For this review, take the finished solid that the model builds, in its own axes (mm). Coordinates: 2 decimals unless noted, no trailing zeros. Loops run counter-clockwise (first coordinate to the right, second up) from the corner with the lowest first, then second, coordinate; pieces in that order, holes last. Notation, with made-up numbers: (4, -30) -> (43, -30) arc R5 ccw to (43, -26) -> close; hole circle Ø2 at (34, -4.5). An arc over 180 degrees is marked (long way). One line per item, written item: value.
from build123d import *

# Parameters (mm, degrees)
SKETCH1_R           = 14.2875
SKETCH1_R_2         = 9.525
SKETCH1_R_3         = 2.4892
BOSS_EXTRUDE3_DEPTH = 3.175


with BuildPart() as part:
    # Sketch1 → Boss-Extrude3 (new body)
    with BuildSketch(Plane.XY):
        Polygon((93.273189322, 200.025), (-25.168955849, -53.975), (-25.168955849, -117.475), (279.631044151, -117.475), (279.631044151, -53.975), (398.073189322, 200.025), align=None)
        with Locations((32.394386098, 20.6375)):
            Circle(SKETCH1_R, mode=Mode.SUBTRACT)
        with Locations((137.394386098, 20.6375)):
            Circle(SKETCH1_R, mode=Mode.SUBTRACT)
        with Locations((242.394386098, 20.6375)):
            Circle(SKETCH1_R, mode=Mode.SUBTRACT)
        with Locations((106.42072683, 179.3875)):
            Circle(SKETCH1_R, mode=Mode.SUBTRACT)
        with Locations((211.39892683, 179.3875)):
            Circle(SKETCH1_R, mode=Mode.SUBTRACT)
        with Locations((189.894386098, -18.746667191)):
            Circle(SKETCH1_R_2, mode=Mode.SUBTRACT)
        with Locations((84.894386098, -21.788906871)):
            Circle(SKETCH1_R_2, mode=Mode.SUBTRACT)
        with Locations((266.931044151, -79.375)):
            Circle(SKETCH1_R_3, mode=Mode.SUBTRACT)
        with Locations((-12.468955849, -104.775)):
            Circle(SKETCH1_R_3, mode=Mode.SUBTRACT)
        with Locations((0.231044151, -104.775)):
            Circle(SKETCH1_R_3, mode=Mode.SUBTRACT)
        with Locations((12.931044151, -104.775)):
            Circle(SKETCH1_R_3, mode=Mode.SUBTRACT)
        with Locations((25.631044151, -104.775)):
            Circle(SKETCH1_R_3, mode=Mode.SUBTRACT)
        with Locations((-12.468955849, -92.075)):
            Circle(SKETCH1_R_3, mode=Mode.SUBTRACT)
        with Locations((0.231044151, -92.075)):
            Circle(SKETCH1_R_3, mode=Mode.SUBTRACT)
        with Locations((-12.468955849, -79.375)):
            Circle(SKETCH1_R_3, mode=Mode.SUBTRACT)
        with Locations((0.231044151, -79.375)):
            Circle(SKETCH1_R_3, mode=Mode.SUBTRACT)
        with Locations((12.931044151, -92.075)):
            Circle(SKETCH1_R_3, mode=Mode.SUBTRACT)
        with Locations((25.631044151, -92.075)):
            Circle(SKETCH1_R_3, mode=Mode.SUBTRACT)
        with Locations((12.931044151, -79.375)):
            Circle(SKETCH1_R_3, mode=Mode.SUBTRACT)
        with Locations((25.631044151, -79.375)):
            Circle(SKETCH1_R_3, mode=Mode.SUBTRACT)
        with Locations((38.331044151, -104.775)):
            Circle(SKETCH1_R_3, mode=Mode.SUBTRACT)
        with Locations((51.031044151, -104.775)):
            Circle(SKETCH1_R_3, mode=Mode.SUBTRACT)
        with Locations((63.731044151, -104.775)):
            Circle(SKETCH1_R_3, mode=Mode.SUBTRACT)
        with Locations((76.431044151, -104.775)):
            Circle(SKETCH1_R_3, mode=Mode.SUBTRACT)
        with Locations((38.331044151, -92.075)):
            Circle(SKETCH1_R_3, mode=Mode.SUBTRACT)
        with Locations((51.031044151, -92.075)):
            Circle(SKETCH1_R_3, mode=Mode.SUBTRACT)
        with Locations((38.331044151, -79.375)):
            Circle(SKETCH1_R_3, mode=Mode.SUBTRACT)
        with Locations((51.031044151, -79.375)):
            Circle(SKETCH1_R_3, mode=Mode.SUBTRACT)
        with Locations((63.731044151, -92.075)):
            Circle(SKETCH1_R_3, mode=Mode.SUBTRACT)
        with Locations((76.431044151, -92.075)):
            Circle(SKETCH1_R_3, mode=Mode.SUBTRACT)
        with Locations((63.731044151, -79.375)):
            Circle(SKETCH1_R_3, mode=Mode.SUBTRACT)
        with Locations((76.431044151, -79.375)):
            Circle(SKETCH1_R_3, mode=Mode.SUBTRACT)
        with Locations((89.131044151, -104.775)):
            Circle(SKETCH1_R_3, mode=Mode.SUBTRACT)
        with Locations((101.831044151, -104.775)):
            Circle(SKETCH1_R_3, mode=Mode.SUBTRACT)
        with Locations((114.531044151, -104.775)):
            Circle(SKETCH1_R_3, mode=Mode.SUBTRACT)
        with Locations((127.231044151, -104.775)):
            Circle(SKETCH1_R_3, mode=Mode.SUBTRACT)
        with Locations((89.131044151, -92.075)):
            Circle(SKETCH1_R_3, mode=Mode.SUBTRACT)
        with Locations((101.831044151, -92.075)):
            Circle(SKETCH1_R_3, mode=Mode.SUBTRACT)
        with Locations((89.131044151, -79.375)):
            Circle(SKETCH1_R_3, mode=Mode.SUBTRACT)
        with Locations((101.831044151, -79.375)):
            Circle(SKETCH1_R_3, mode=Mode.SUBTRACT)
        with Locations((114.531044151, -92.075)):
            Circle(SKETCH1_R_3, mode=Mode.SUBTRACT)
        with Locations((127.231044151, -92.075)):
            Circle(SKETCH1_R_3, mode=Mode.SUBTRACT)
        with Locations((114.531044151, -79.375)):
            Circle(SKETCH1_R_3, mode=Mode.SUBTRACT)
        with Locations((127.231044151, -79.375)):
            Circle(SKETCH1_R_3, mode=Mode.SUBTRACT)
        with Locations((139.931044151, -104.775)):
            Circle(SKETCH1_R_3, mode=Mode.SUBTRACT)
        with Locations((152.631044151, -104.775)):
            Circle(SKETCH1_R_3, mode=Mode.SUBTRACT)
        with Locations((165.331044151, -104.775)):
            Circle(SKETCH1_R_3, mode=Mode.SUBTRACT)
        with Locations((178.031044151, -104.775)):
            Circle(SKETCH1_R_3, mode=Mode.SUBTRACT)
        with Locations((139.931044151, -92.075)):
            Circle(SKETCH1_R_3, mode=Mode.SUBTRACT)
        with Locations((152.631044151, -92.075)):
            Circle(SKETCH1_R_3, mode=Mode.SUBTRACT)
        with Locations((139.931044151, -79.375)):
            Circle(SKETCH1_R_3, mode=Mode.SUBTRACT)
        with Locations((152.631044151, -79.375)):
            Circle(SKETCH1_R_3, mode=Mode.SUBTRACT)
        with Locations((165.331044151, -92.075)):
            Circle(SKETCH1_R_3, mode=Mode.SUBTRACT)
        with Locations((178.031044151, -92.075)):
            Circle(SKETCH1_R_3, mode=Mode.SUBTRACT)
        with Locations((165.331044151, -79.375)):
            Circle(SKETCH1_R_3, mode=Mode.SUBTRACT)
        with Locations((178.031044151, -79.375)):
            Circle(SKETCH1_R_3, mode=Mode.SUBTRACT)
        with Locations((190.731044151, -104.775)):
            Circle(SKETCH1_R_3, mode=Mode.SUBTRACT)
        with Locations((203.431044151, -104.775)):
            Circle(SKETCH1_R_3, mode=Mode.SUBTRACT)
        with Locations((216.131044151, -104.775)):
            Circle(SKETCH1_R_3, mode=Mode.SUBTRACT)
        with Locations((228.831044151, -104.775)):
            Circle(SKETCH1_R_3, mode=Mode.SUBTRACT)
        with Locations((190.731044151, -92.075)):
            Circle(SKETCH1_R_3, mode=Mode.SUBTRACT)
        with Locations((203.431044151, -92.075)):
            Circle(SKETCH1_R_3, mode=Mode.SUBTRACT)
        with Locations((190.731044151, -79.375)):
            Circle(SKETCH1_R_3, mode=Mode.SUBTRACT)
        with Locations((203.431044151, -79.375)):
            Circle(SKETCH1_R_3, mode=Mode.SUBTRACT)
        with Locations((216.131044151, -92.075)):
            Circle(SKETCH1_R_3, mode=Mode.SUBTRACT)
        with Locations((228.831044151, -92.075)):
            Circle(SKETCH1_R_3, mode=Mode.SUBTRACT)
        with Locations((216.131044151, -79.375)):
            Circle(SKETCH1_R_3, mode=Mode.SUBTRACT)
        with Locations((228.831044151, -79.375)):
            Circle(SKETCH1_R_3, mode=Mode.SUBTRACT)
        with Locations((241.531044151, -104.775)):
            Circle(SKETCH1_R_3, mode=Mode.SUBTRACT)
        with Locations((254.231044151, -104.775)):
            Circle(SKETCH1_R_3, mode=Mode.SUBTRACT)
        with Locations((266.931044151, -104.775)):
            Circle(SKETCH1_R_3, mode=Mode.SUBTRACT)
        with Locations((241.531044151, -92.075)):
            Circle(SKETCH1_R_3, mode=Mode.SUBTRACT)
        with Locations((254.231044151, -92.075)):
            Circle(SKETCH1_R_3, mode=Mode.SUBTRACT)
        with Locations((241.531044151, -79.375)):
            Circle(SKETCH1_R_3, mode=Mode.SUBTRACT)
        with Locations((254.231044151, -79.375)):
            Circle(SKETCH1_R_3, mode=Mode.SUBTRACT)
        with Locations((266.931044151, -92.075)):
            Circle(SKETCH1_R_3, mode=Mode.SUBTRACT)
    extrude(amount=BOSS_EXTRUDE3_DEPTH)


solid = part.part
1. Take a section at C-C, the plane z = 0.55. Give the number of separate pieces and of enclosed holes in the cut face, and give its area (3 significant figures).
Return value:
separate pieces: 1
enclosed holes: 76
area: 91,700 mm2
2. To check wall thickness, follow probe 1 along Y at (x, z) = (178, 0.7) (3 decimals); probe 2 along Y at (x, z) = (78, 1.15) (3 decimals); probe 3 along Y at (x, z) = (13.5, 2.95) (3 decimals). State the ranges of each line that lie inside material, in increasing order. Write a range as from..to.
Return value:
probe 1: y = -117.475..-107.264, -102.286..-94.564, -89.586..-81.864, -76.886..200.025
probe 2: y = -117.475..-106.707, -102.843..-94.007, -90.143..-81.307, -77.443..-28.361, -15.217..167.272
probe 3: y = -117.475..-107.198, -102.352..-94.498, -89.652..-81.798, -76.952..28.951
3. Take a section at D-D, the plane y = 89.5. Give the boundary of the cut face in (x, z) (3 decimals), and give its area (3 significant figures).
Return value:
outline: (41.735, 0) -> (346.535, 0) -> (346.535, 3.175) -> (41.735, 3.175) -> close
area: 968 mm2
4. The part is to be moulded in two halves that separate along X. For faces 1 (the flat face through (183, 43, 0)), 2 (the cylindrical face through (94, -19, 2)), 3 (the flat face through (34.88, 74.8, 1.57)), say which applies: pulls with the +X half, pulls with the -X half, needs draft (parallel to the pull), parting line crosses it, or undercut.
Return value:
face 1: needs draft
face 2: undercut
face 3: pulls with the -X half
5. Insertion check: pin 1 Ø4 at (x, y) = (152.63, -92.08) entering from -Z; pin 2 Ø1 at (y, z) = (99, 0.5) entering from -X. Each pin has a flat end and moves straight along its axis. Give the tip position at first contact, or say it passes through.
Return value:
pin 1: passes through
pin 2: stops at x = 45.93
6. Take a section at A-A, the plane y = 11.5. Give the boundary of the cut face in (x, z) (3 decimals), and give its area (3 significant figures).
Return value:
outline: (5.363, 0) -> (21.411, 0) -> (21.411, 3.175) -> (5.363, 3.175) -> close; (43.378, 0) -> (126.411, 0) -> (126.411, 3.175) -> (43.378, 3.175) -> close; (148.378, 0) -> (231.411, 0) -> (231.411, 3.175) -> (148.378, 3.175) -> close; (253.378, 0) -> (310.163, 0) -> (310.163, 3.175) -> (253.378, 3.175) -> close
area: 759 mm2
7. Take a section at B-B, the plane x = 311.5. Give the boundary of the cut face in (y, z) (3 decimals).
Return value:
outline: (14.368, 0) -> (200.025, 0) -> (200.025, 3.175) -> (14.368, 3.175) -> close
